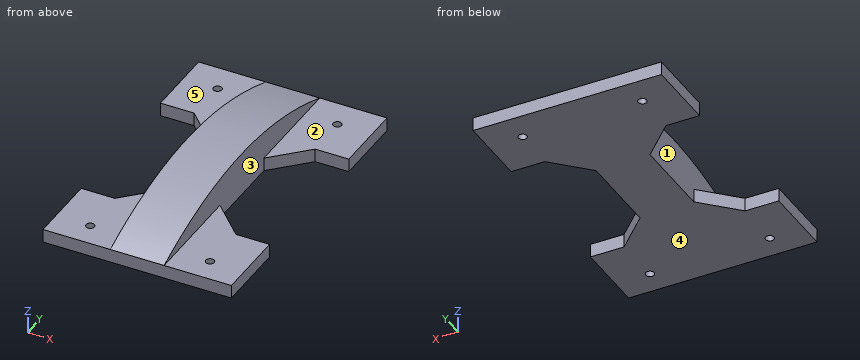
from build123d import *

# Parameters (mm, degrees)
SKETCH_1_W          = 70
SKETCH_1_H          = 110
EXTRUDE_1_DEPTH     = 5
SKETCH_2_R          = 1.57
CUT_EXTRUDE_1_DEPTH = 5
CUT_EXTRUDE_2_DEPTH = 5
EXTRUDE_START       = -20
EXTRUDE_3_DEPTH     = 20


with BuildPart() as part:
    # 草图1 → 凸台-拉伸1 (new body)
    with BuildSketch(Plane.XY):
        with Locations((-7.671321449, -10.342578999)):
            Rectangle(SKETCH_1_W, SKETCH_1_H)
    extrude(amount=EXTRUDE_1_DEPTH)

    # 草图2 → 切除-拉伸1 (cut)
    with BuildSketch(Plane.XY.offset(5)):
        with Locations((-29.921321449, 33.811245296)):
            Circle(SKETCH_2_R)
        with Locations((14.578678551, 33.811245296)):
            Circle(SKETCH_2_R)
        with Locations((-29.921321449, -56.188754704)):
            Circle(SKETCH_2_R)
        with Locations((14.578678551, -56.188754704)):
            Circle(SKETCH_2_R)
    extrude(amount=-CUT_EXTRUDE_1_DEPTH, mode=Mode.SUBTRACT)

    # 草图3 → 切除-拉伸2 (cut)
    with BuildSketch(Plane.XY.offset(5)):
        Polygon((-42.671321449, 17.657421001), (-30.171321449, 17.657421001), (-17.671321449, 5.157421001), (-17.671321449, -25.842578999), (-30.171321449, -38.342578999), (-42.671321449, -38.342578999), align=None)
        Polygon((14.828678551, 17.657421001), (27.328678551, 17.657421001), (27.328678551, -38.342578999), (14.828678551, -38.342578999), (2.328678551, -25.842578999), (2.328678551, 5.157421001), align=None)
    extrude(amount=-CUT_EXTRUDE_2_DEPTH, mode=Mode.SUBTRACT)

    # 草图6 → 凸台-拉伸3 (add)
    with BuildSketch(Plane(origin=(2.328678551, 0, 0), x_dir=(0, 0, -1), z_dir=(1, 0, 0)).offset(EXTRUDE_START)):
        with BuildLine():
            Line((-5, 44.657421001), (-5, -65.342578999))
            add(Edge.make_bspline(
                [(-5, 44.657421001), (-27.43165177, -11.855516643), (-5, -65.342578999)],
                knots=[0, 0, 0, 1, 1, 1], degree=2))
        make_face()
    extrude(amount=EXTRUDE_3_DEPTH)


solid = part.part
Input: part model. Units: mm. Frame: model coordinates. Face numbers are marked on the shaded views. A direction names the side the tool comes from. Give positions to 0.01 mm unless a question says otherwise; leave off trailing zeros. Order: outer loops, then holes, each group sorted by start corner. A loop starts at its lowest first (then second) coordinate and runs counter-clockwise, first axis right, second up.
Q1. Section A-A on x = -33.5. Output: boundary loops of the cut face in (y, z).
Checked values:
outline: (-65.34, 0) - (-38.34, 0) - (-38.34, 5) - (-65.34, 5) - close; (17.66, 0) - (44.66, 0) - (44.66, 5) - (17.66, 5) - close
Q2. Set-up query: the marked faces 1, 2, 3, 4 and 5. Return all of +Z, -Z, +X, -X, +Y, -Y with unobstructed straight access to the full face (end or side cutting, diameter ignored); none if empty.
Checked values:
face 1: +Z, -X
face 2: +Z, +X, +Y, -Y
face 3: +Z, +X
face 4: -Z, +X, -X, +Y, -Y
face 5: +Z, -X, +Y, -Y
Q3. Ray query, probe 1 along X at (y, z) = (9, 11.5); probe 2 along Y at (x, z) = (-38.5, 4.25); probe 3 along Z at (x, y) = (8, 15). Return the intervals inside material, ascending.
Checked values:
probe 1: x = -17.67 to 2.33
probe 2: y = -65.34 to -38.34, 17.66 to 44.66
probe 3: z = 0 to 5
Q4. Section B-B on x = 4. Output: boundary loops of the cut face in (y, z), and give its area (3 significant figures).
Checked values:
outline: (-65.34, 0) - (-27.51, 0) - (-27.51, 5) - (-65.34, 5) - close; (6.83, 0) - (44.66, 0) - (44.66, 5) - (6.83, 5) - close
area: 378 mm2
Q5. Contact query for flat-ended pins moving along their axis: pin 1 Ø5 at (y, z) = (-14, 4) entering from -X; pin 2 Ø20 at (x, y) = (15.5, 19) entering from +Z; pin 3 Ø6 at (y, z) = (2.5, 8) entering from +X. Output: stop coordinate, or through.
Checked values:
pin 1: stops at x = -17.67
pin 2: stops at z = 5
pin 3: stops at x = 2.33
